Geometry: final body of the model. Coordinates: model frame, mm. A direction names the side the tool comes from. Round coordinates to 2 decimals unless told otherwise and drop trailing zeros. Loops run counter-clockwise (first coordinate to the right, second up) from the corner with the lowest first, then second, coordinate; pieces in that order, holes last. Notation, with made-up numbers: (6.25, -20) - (27.25, -20) arc R23 ccw to (27.25, 17) - close; hole circle Ø5 at (-14.5, 46). An arc over 180 degrees is marked (long way). Use CSV: the item, a comma, the result in double quotes.
from build123d import *

# Parameters (mm, degrees)
BOSS_EXTRUDE1_DEPTH = 37
CUT_EXTRUDE1_REACH  = 152.396
SKETCH2_R           = 11.5
CUT_EXTRUDE2_REACH  = 152.396
SKETCH3_R           = 1.25
CUT_EXTRUDE5_REACH  = 152.396
SKETCH5_R           = 1.25
BOSS_EXTRUDE3_START = 6
SKETCH6_R           = 11
SKETCH6_R_2         = 1.25
BOSS_EXTRUDE3_DEPTH = 6
SKETCH4_W           = 38
SKETCH4_H           = 23
CUT_EXTRUDE6_DEPTH  = 3
SKETCH9_R           = 2.05
CUT_EXTRUDE8_DEPTH  = 2
SKETCH10_R          = 2.55
CUT_EXTRUDE9_DEPTH  = 6
CHAMFER1_SIZE       = 20
FILLET5_R           = 10
CUT_EXTRUDE10_REACH = 148.571
SKETCH11_R          = 1.25
SKETCH12_R          = 2.05
CUT_EXTRUDE11_DEPTH = 2
SKETCH7_W           = 3
SKETCH7_H           = 23
BOSS_EXTRUDE4_DEPTH = 0.5


with BuildPart() as part:
    # Sketch1 → Boss-Extrude1 (new body)
    with BuildSketch(Plane(origin=(0, 0, 0), x_dir=(1, 0, 0), z_dir=(0, 1, 0))):
        Polygon((0, 0), (0, 75), (125, 75), (125, 67), (8, 67), (8, 0), align=None)
    extrude(amount=BOSS_EXTRUDE1_DEPTH)

    # Sketch2 → Cut-Extrude1 (cut, up to next)
    with BuildSketch(Plane(origin=(0, 0, -75), x_dir=(-1, 0, 0), z_dir=(0, 0, -1)), mode=Mode.PRIVATE) as cut_extrude1_sk1:
        with Locations((-109, 18.5)):
            Circle(SKETCH2_R)
    cut_extrude1_tool1 = extrude(cut_extrude1_sk1.sketch, amount=-CUT_EXTRUDE1_REACH, mode=Mode.PRIVATE) & part.part
    add(cut_extrude1_tool1.solids().sort_by_distance((109, 18.5, -75))[0], mode=Mode.SUBTRACT)

    # Sketch3 → Cut-Extrude2 (cut, up to next)
    with BuildSketch(Plane(origin=(0, 0, -75), x_dir=(-1, 0, 0), z_dir=(0, 0, -1)), mode=Mode.PRIVATE) as cut_extrude2_sk1:
        with Locations((-102.36, 32.19)):
            Circle(SKETCH3_R)
    cut_extrude2_tool1 = extrude(cut_extrude2_sk1.sketch, amount=-CUT_EXTRUDE2_REACH, mode=Mode.PRIVATE) & part.part
    # Sketch3 → Cut-Extrude2 (cut, up to next)
    with BuildSketch(Plane(origin=(0, 0, -75), x_dir=(-1, 0, 0), z_dir=(0, 0, -1)), mode=Mode.PRIVATE) as cut_extrude2_sk2:
        with Locations((-94.36, 32.19)):
            Circle(SKETCH3_R)
    cut_extrude2_tool2 = extrude(cut_extrude2_sk2.sketch, amount=-CUT_EXTRUDE2_REACH, mode=Mode.PRIVATE) & part.part
    # Sketch3 → Cut-Extrude2 (cut, up to next)
    with BuildSketch(Plane(origin=(0, 0, -75), x_dir=(-1, 0, 0), z_dir=(0, 0, -1)), mode=Mode.PRIVATE) as cut_extrude2_sk3:
        with Locations((-86.36, 32.19)):
            Circle(SKETCH3_R)
    cut_extrude2_tool3 = extrude(cut_extrude2_sk3.sketch, amount=-CUT_EXTRUDE2_REACH, mode=Mode.PRIVATE) & part.part
    # Sketch3 → Cut-Extrude2 (cut, up to next)
    with BuildSketch(Plane(origin=(0, 0, -75), x_dir=(-1, 0, 0), z_dir=(0, 0, -1)), mode=Mode.PRIVATE) as cut_extrude2_sk4:
        with Locations((-78.36, 32.19)):
            Circle(SKETCH3_R)
    cut_extrude2_tool4 = extrude(cut_extrude2_sk4.sketch, amount=-CUT_EXTRUDE2_REACH, mode=Mode.PRIVATE) & part.part
    # Sketch3 → Cut-Extrude2 (cut, up to next)
    with BuildSketch(Plane(origin=(0, 0, -75), x_dir=(-1, 0, 0), z_dir=(0, 0, -1)), mode=Mode.PRIVATE) as cut_extrude2_sk5:
        with Locations((-78.36, 4.81)):
            Circle(SKETCH3_R)
    cut_extrude2_tool5 = extrude(cut_extrude2_sk5.sketch, amount=-CUT_EXTRUDE2_REACH, mode=Mode.PRIVATE) & part.part
    # Sketch3 → Cut-Extrude2 (cut, up to next)
    with BuildSketch(Plane(origin=(0, 0, -75), x_dir=(-1, 0, 0), z_dir=(0, 0, -1)), mode=Mode.PRIVATE) as cut_extrude2_sk6:
        with Locations((-86.36, 4.81)):
            Circle(SKETCH3_R)
    cut_extrude2_tool6 = extrude(cut_extrude2_sk6.sketch, amount=-CUT_EXTRUDE2_REACH, mode=Mode.PRIVATE) & part.part
    # Sketch3 → Cut-Extrude2 (cut, up to next)
    with BuildSketch(Plane(origin=(0, 0, -75), x_dir=(-1, 0, 0), z_dir=(0, 0, -1)), mode=Mode.PRIVATE) as cut_extrude2_sk7:
        with Locations((-94.36, 4.81)):
            Circle(SKETCH3_R)
    cut_extrude2_tool7 = extrude(cut_extrude2_sk7.sketch, amount=-CUT_EXTRUDE2_REACH, mode=Mode.PRIVATE) & part.part
    # Sketch3 → Cut-Extrude2 (cut, up to next)
    with BuildSketch(Plane(origin=(0, 0, -75), x_dir=(-1, 0, 0), z_dir=(0, 0, -1)), mode=Mode.PRIVATE) as cut_extrude2_sk8:
        with Locations((-102.36, 4.81)):
            Circle(SKETCH3_R)
    cut_extrude2_tool8 = extrude(cut_extrude2_sk8.sketch, amount=-CUT_EXTRUDE2_REACH, mode=Mode.PRIVATE) & part.part
    add(cut_extrude2_tool1.solids().sort_by_distance((102.36, 32.19, -75))[0], mode=Mode.SUBTRACT)
    add(cut_extrude2_tool2.solids().sort_by_distance((94.36, 32.19, -75))[0], mode=Mode.SUBTRACT)
    add(cut_extrude2_tool3.solids().sort_by_distance((86.36, 32.19, -75))[0], mode=Mode.SUBTRACT)
    add(cut_extrude2_tool4.solids().sort_by_distance((78.36, 32.19, -75))[0], mode=Mode.SUBTRACT)
    add(cut_extrude2_tool5.solids().sort_by_distance((78.36, 4.81, -75))[0], mode=Mode.SUBTRACT)
    add(cut_extrude2_tool6.solids().sort_by_distance((86.36, 4.81, -75))[0], mode=Mode.SUBTRACT)
    add(cut_extrude2_tool7.solids().sort_by_distance((94.36, 4.81, -75))[0], mode=Mode.SUBTRACT)
    add(cut_extrude2_tool8.solids().sort_by_distance((102.36, 4.81, -75))[0], mode=Mode.SUBTRACT)

    # Sketch5 → Cut-Extrude5 (cut, up to next)
    with BuildSketch(Plane.ZY, mode=Mode.PRIVATE) as cut_extrude5_sk1:
        with Locations((-16, 10.5)):
            Circle(SKETCH5_R)
    cut_extrude5_tool1 = extrude(cut_extrude5_sk1.sketch, amount=-CUT_EXTRUDE5_REACH, mode=Mode.PRIVATE) & part.part
    # Sketch5 → Cut-Extrude5 (cut, up to next)
    with BuildSketch(Plane.ZY, mode=Mode.PRIVATE) as cut_extrude5_sk2:
        with Locations((-24, 18.5)):
            Circle(SKETCH5_R)
    cut_extrude5_tool2 = extrude(cut_extrude5_sk2.sketch, amount=-CUT_EXTRUDE5_REACH, mode=Mode.PRIVATE) & part.part
    # Sketch5 → Cut-Extrude5 (cut, up to next)
    with BuildSketch(Plane.ZY, mode=Mode.PRIVATE) as cut_extrude5_sk3:
        with Locations((-16, 26.5)):
            Circle(SKETCH5_R)
    cut_extrude5_tool3 = extrude(cut_extrude5_sk3.sketch, amount=-CUT_EXTRUDE5_REACH, mode=Mode.PRIVATE) & part.part
    # Sketch5 → Cut-Extrude5 (cut, up to next)
    with BuildSketch(Plane.ZY, mode=Mode.PRIVATE) as cut_extrude5_sk4:
        with Locations((-8, 18.5)):
            Circle(SKETCH5_R)
    cut_extrude5_tool4 = extrude(cut_extrude5_sk4.sketch, amount=-CUT_EXTRUDE5_REACH, mode=Mode.PRIVATE) & part.part
    add(cut_extrude5_tool1.solids().sort_by_distance((0, 10.5, -16))[0], mode=Mode.SUBTRACT)
    add(cut_extrude5_tool2.solids().sort_by_distance((0, 18.5, -24))[0], mode=Mode.SUBTRACT)
    add(cut_extrude5_tool3.solids().sort_by_distance((0, 26.5, -16))[0], mode=Mode.SUBTRACT)
    add(cut_extrude5_tool4.solids().sort_by_distance((0, 18.5, -8))[0], mode=Mode.SUBTRACT)

    # Sketch6 → Boss-Extrude3 (add)
    with BuildSketch(Plane.ZY.offset(BOSS_EXTRUDE3_START)):
        with Locations(Location((-16, 18.5, 0), (0, 0, 180))):
            Circle(SKETCH6_R)
        with Locations((-16, 10.5)):
            Circle(SKETCH6_R_2, mode=Mode.SUBTRACT)
        with Locations((-24, 18.5)):
            Circle(SKETCH6_R_2, mode=Mode.SUBTRACT)
        with Locations((-16, 26.5)):
            Circle(SKETCH6_R_2, mode=Mode.SUBTRACT)
        with Locations((-8, 18.5)):
            Circle(SKETCH6_R_2, mode=Mode.SUBTRACT)
    extrude(amount=-BOSS_EXTRUDE3_DEPTH)

    # Sketch4 → Cut-Extrude6 (cut)
    with BuildSketch(Plane(origin=(0, 0, -75), x_dir=(-1, 0, 0), z_dir=(0, 0, -1))):
        with Locations((-94, 18.5)):
            Rectangle(SKETCH4_W, SKETCH4_H)
    extrude(amount=-CUT_EXTRUDE6_DEPTH, mode=Mode.SUBTRACT)

    # Sketch9 → Cut-Extrude8 (cut)
    with BuildSketch(Plane.XY.offset(-67)):
        with Locations((78.36, 32.19)):
            Circle(SKETCH9_R)
        with Locations((86.36, 32.19)):
            Circle(SKETCH9_R)
        with Locations((94.36, 32.19)):
            Circle(SKETCH9_R)
        with Locations((102.36, 32.19)):
            Circle(SKETCH9_R)
        with Locations((78.36, 4.81)):
            Circle(SKETCH9_R)
        with Locations((86.36, 4.81)):
            Circle(SKETCH9_R)
        with Locations((94.36, 4.81)):
            Circle(SKETCH9_R)
        with Locations((102.36, 4.81)):
            Circle(SKETCH9_R)
    extrude(amount=-CUT_EXTRUDE8_DEPTH, mode=Mode.SUBTRACT)

    # Sketch10 → Cut-Extrude9 (cut)
    with BuildSketch(Plane(origin=(8, 0, 0), x_dir=(0, 0, -1), z_dir=(1, 0, 0))):
        with Locations((24, 18.5)):
            Circle(SKETCH10_R)
        with Locations((16, 10.5)):
            Circle(SKETCH10_R)
        with Locations((8, 18.5)):
            Circle(SKETCH10_R)
        with Locations((16, 26.5)):
            Circle(SKETCH10_R)
    extrude(amount=-CUT_EXTRUDE9_DEPTH, mode=Mode.SUBTRACT)

    # Chamfer1
    chamfer1_edges = [part.edges().sort_by_distance(p)[0] for p in [
        (8, 18.5, -67),
    ]]
    chamfer(chamfer1_edges, length=CHAMFER1_SIZE)

    # Fillet5
    fillet5_edges = [part.edges().sort_by_distance(p)[0] for p in [
        (28, 18.5, -67),
        (8, 18.5, -47),
    ]]
    fillet(fillet5_edges, radius=FILLET5_R)

    # Sketch11 → Cut-Extrude10 (cut, up to next)
    with BuildSketch(Plane.XY.offset(-67), mode=Mode.PRIVATE) as cut_extrude10_sk1:
        with Locations((72.86, 10.31)):
            Circle(SKETCH11_R)
    cut_extrude10_tool1 = extrude(cut_extrude10_sk1.sketch, amount=-CUT_EXTRUDE10_REACH, mode=Mode.PRIVATE) & part.part
    # Sketch11 → Cut-Extrude10 (cut, up to next)
    with BuildSketch(Plane.XY.offset(-67), mode=Mode.PRIVATE) as cut_extrude10_sk2:
        with Locations((72.86, 26.69)):
            Circle(SKETCH11_R)
    cut_extrude10_tool2 = extrude(cut_extrude10_sk2.sketch, amount=-CUT_EXTRUDE10_REACH, mode=Mode.PRIVATE) & part.part
    add(cut_extrude10_tool1.solids().sort_by_distance((72.86, 10.31, -67))[0], mode=Mode.SUBTRACT)
    add(cut_extrude10_tool2.solids().sort_by_distance((72.86, 26.69, -67))[0], mode=Mode.SUBTRACT)

    # Sketch12 → Cut-Extrude11 (cut)
    with BuildSketch(Plane.XY.offset(-67)):
        with Locations((72.86, 10.31)):
            Circle(SKETCH12_R)
        with Locations((72.86, 26.69)):
            Circle(SKETCH12_R)
    extrude(amount=-CUT_EXTRUDE11_DEPTH, mode=Mode.SUBTRACT)

    # Sketch7 → Boss-Extrude4 (add)
    with BuildSketch(Plane(origin=(75, 0, 0), x_dir=(0, 0, -1), z_dir=(1, 0, 0))):
        with Locations((73.5, 18.5)):
            Rectangle(SKETCH7_W, SKETCH7_H)
    extrude(amount=BOSS_EXTRUDE4_DEPTH)


solid = part.part
Item 1: Section C-C on y = 18.5. Give the number of separate pieces and of enclosed holes in the cut face, plus the area to 3 significant figures.
Final values:
separate pieces,"4"
enclosed holes,"0"
area,"1,520 mm²"
Item 2: Section B-B on z = -8. Return the cut outline in (x, y), plus the area to 3 significant figures.
Final values:
outline,"(-6, 10.95) - (0, 10.95) - (0, 0) - (8, 0) - (8, 15.95) - (2, 15.95) - (2, 17.25) - (-6, 17.25) - close; (-6, 19.75) - (2, 19.75) - (2, 21.05) - (8, 21.05) - (8, 37) - (0, 37) - (0, 26.05) - (-6, 26.05) - close"
area,"336 mm²"
Item 3: Mould query, pull axis Y, two halves, no side actions, for faces 5 (the cylindrical face through (70.81, 10.4, -67.99)), 6 (the cylindrical face through (-3.04, 29.24, -13.62)), 7 (the cylindrical face through (8.782, 18.759, -46.735)). Classes: released by +Y, released by -Y, zero draft, split by the parting line, or undercut.
Final values:
face 5,"undercut"
face 6,"split by the parting line"
face 7,"zero draft"
Item 4: Reachability of faces 1 (the cylindrical face through (-2.056, 18.021, -22.845)), 2 (the cylindrical face through (76.849, 33.575, -67.986)), 3 (the flat face through (2, 9, -15)), 4 (the flat face through (75.5, 19, -73)) from +Z, -Z, +X, -X, +Y, -Y: full face, straight path, thin tool, end or side. Return the list, or none.
Final values:
face 1,"+X, -X"
face 2,"+Z"
face 3,"+X"
face 4,"-Z"
Item 5: Material intervals for line 1 (Y direction, x = 102.36, z = -72.9); line 2 (Y direction, x = 4, z = -16); line 3 (Y direction, x = 4, z = -24), sorted ascending.
Final values:
line 1,"y = 0 to 3.56, 6.06 to 7, 30 to 30.94, 33.44 to 37"
line 2,"y = 0 to 7.95, 13.05 to 23.95, 29.05 to 37"
line 3,"y = 0 to 15.95, 21.05 to 37"
Item 6: Section D-D on z = -62.5. Return the cut outline in (x, y), plus the area to 4 significant figures.
Final values:
outline,"(0, 0) - (23.5, 0) - (23.5, 37) - (0, 37) - close"
area,"869.5 mm²"
Item 7: Pin query (flat end, axial travel): P1, Ø2, axis at y = 25.5, z = -34, coming from the +X side; P2, Ø4.5, axis at x = 79, y = 33, coming from the +Z side; P3, Ø6, axis at y = 25.5, z = -29.5, coming from the -X side; P4, Ø2, axis at x = 102.36, y = 4.81, coming from the -Z side. Return the tip coordinate at first contact, or that it passes through.
Final values:
P1,"stops at x = 8"
P2,"stops at z = -67"
P3,"stops at x = 0"
P4,"passes through"
Item 8: Section A-A on x = 94.36. Return the cut outline in (y, z), plus the area to 3 significant figures.
Final values:
outline,"(0, -75) - (3.56, -75) - (3.56, -69) - (2.76, -69) - (2.76, -67) - (0, -67) - close; (6.06, -75) - (7, -75) - (7, -72) - (30, -72) - (30, -75) - (30.94, -75) - (30.94, -69) - (30.14, -69) - (30.14, -67) - (6.86, -67) - (6.86, -69) - (6.06, -69) - close; (33.44, -75) - (37, -75) - (37, -67) - (34.24, -67) - (34.24, -69) - (33.44, -69) - close"
area,"181 mm²"
